Autodesk Inventor part; units mm, degrees
ref_plane "YZ Plane" through (0, 0, 0) normal (1, 0, 0) x (0, 1, 0)
ref_plane "XZ Plane" through (0, 0, 0) normal (0, 1, 0) x (-1, 0, 0)
ref_plane "XY Plane" through (0, 0, 0) normal (0, 0, 1) x (1, 0, 0)
sketch "Foam Scheme" plane through (0, 0, 0) normal (0, 1, 0) x (-1, 0, 0)
  line L0 (929.5, -94) -> (-929.5, -94)
  line L1 (-929.5, -94) -> (-929.5, 94)
  line L2 (-929.5, 94) -> (929.5, 94)
  line L3 (929.5, 94) -> (929.5, -94)
  circle A0 centre (907.5, -72) radius 9.5
  circle A1 centre (852.5, -72) radius 9.5
  circle A2 centre (797.5, -72) radius 9.5
  circle A3 centre (742.5, -72) radius 9.5
  circle A4 centre (687.5, -72) radius 9.5
  circle A5 centre (632.5, -72) radius 9.5
  circle A6 centre (577.5, -72) radius 9.5
  circle A7 centre (522.5, -72) radius 9.5
  circle A8 centre (467.5, -72) radius 9.5
  circle A9 centre (412.5, -72) radius 9.5
  circle A10 centre (357.5, -72) radius 9.5
  circle A11 centre (302.5, -72) radius 9.5
  circle A12 centre (247.5, -72) radius 9.5
  circle A13 centre (192.5, -72) radius 9.5
  circle A14 centre (137.5, -72) radius 9.5
  circle A15 centre (82.5, -72) radius 9.5
  circle A16 centre (27.5, -72) radius 9.5
  circle A17 centre (-27.5, -72) radius 9.5
  circle A18 centre (907.5, 72) radius 9.5
  circle A19 centre (852.5, 72) radius 9.5
  circle A20 centre (797.5, 72) radius 9.5
  circle A21 centre (742.5, 72) radius 9.5
  circle A22 centre (687.5, 72) radius 9.5
  circle A23 centre (632.5, 72) radius 9.5
  circle A24 centre (577.5, 72) radius 9.5
  circle A25 centre (522.5, 72) radius 9.5
  circle A26 centre (467.5, 72) radius 9.5
  circle A27 centre (412.5, 72) radius 9.5
  circle A28 centre (357.5, 72) radius 9.5
  circle A29 centre (302.5, 72) radius 9.5
  circle A30 centre (247.5, 72) radius 9.5
  circle A31 centre (192.5, 72) radius 9.5
  circle A32 centre (137.5, 72) radius 9.5
  circle A33 centre (82.5, 72) radius 9.5
  circle A34 centre (27.5, 72) radius 9.5
  circle A35 centre (-27.5, 72) radius 9.5
  circle A36 centre (-82.5, -72) radius 9.5
  circle A37 centre (-82.5, 72) radius 9.5
  circle A38 centre (-137.5, -72) radius 9.5
  circle A39 centre (-137.5, 72) radius 9.5
  circle A40 centre (-192.5, -72) radius 9.5
  circle A41 centre (-192.5, 72) radius 9.5
  circle A42 centre (-247.5, -72) radius 9.5
  circle A43 centre (-247.5, 72) radius 9.5
  circle A44 centre (-302.5, -72) radius 9.5
  circle A45 centre (-302.5, 72) radius 9.5
  circle A46 centre (-357.5, -72) radius 9.5
  circle A47 centre (-357.5, 72) radius 9.5
  circle A48 centre (-412.5, -72) radius 9.5
  circle A49 centre (-412.5, 72) radius 9.5
  circle A50 centre (-467.5, -72) radius 9.5
  circle A51 centre (-467.5, 72) radius 9.5
  circle A52 centre (-522.5, -72) radius 9.5
  circle A53 centre (-522.5, 72) radius 9.5
  circle A54 centre (-577.5, -72) radius 9.5
  circle A55 centre (-577.5, 72) radius 9.5
  circle A56 centre (-632.5, -72) radius 9.5
  circle A57 centre (-632.5, 72) radius 9.5
  circle A58 centre (-687.5, -72) radius 9.5
  circle A59 centre (-687.5, 72) radius 9.5
  circle A60 centre (-742.5, -72) radius 9.5
  circle A61 centre (-742.5, 72) radius 9.5
  circle A62 centre (-797.5, -72) radius 9.5
  circle A63 centre (-797.5, 72) radius 9.5
  circle A64 centre (-852.5, -72) radius 9.5
  circle A65 centre (-852.5, 72) radius 9.5
  circle A66 centre (-907.5, -72) radius 9.5
  circle A67 centre (-907.5, 72) radius 9.5
  point P0 (0, 0)
  dimension "d0" = 1859
  dimension "d1" = 929.5
  dimension "d2" = 188
  dimension "d3" = 94
  dimension "d4" = 19
  dimension "d5" = 22
  dimension "d6" = 22
  dimension "d9" = 55
  dimension "d12" = 144
extrude "Foam Body" add sketch "Foam Scheme" along normal blind 1.5
properties part number "Foam NPS 18" material "Rubber, Silicone"
Part model, mm, in its own coordinate system. Round coordinates to 2 decimals unless told otherwise and drop trailing zeros. Use a Markdown table: item, result.
1) Drop a flat-ended pin along its axis: pin 1 Ø11.5 at (x, z) = (-907.5, -72) entering from -Y. Give the stop position or say it passes through.
The answers:
| item | result |
|---|---|
| pin 1 | passes through |
2) Probe line 1 (Z direction, x = 907.5, y = 0.5); line 2 (Z direction, x = -573, y = 0.75). List the from-to ranges inside material, lowest first. Write a range as [from, to].
The answers:
| item | result |
|---|---|
| line 1 | z = [-94, -81.5], [-62.5, 62.5], [81.5, 94] |
| line 2 | z = [-94, -80.37], [-63.63, 63.63], [80.37, 94] |
3) Cut at A-A, the plane y = 0.6. State how many separate pieces and enclosed holes the cut face has, and give its area (3 significant figures).
The answers:
| item | result |
|---|---|
| separate pieces | 1 |
| enclosed holes | 68 |
| area | 330,000 mm2 |
